Job drawing, mm, ordinate dimensions from the low corner. One solid piece. A direction names the side the tool comes from. Coordinates: 2 decimals unless noted, no trailing zeros. Loops run counter-clockwise (first coordinate to the right, second up) from the corner with the lowest first, then second, coordinate; pieces in that order, holes last. Notation, with made-up numbers: (22, -14) - (53, -14) arc R20 ccw to (53, 23) - close; hole circle Ø1 at (7, 36.25). An arc over 180 degrees is marked (long way). Use a Markdown table: item, result. Add a question column.
1. Band-saw the part on B-B, the plane z = 3.75. Give the cut face in (x, y) (1 decimal), plus the area to 3 significant figures.
2. Band-saw the part on C-C, the plane x = 20.25. Give the cut face in (y, z).
3. Wall check: probe 1 along X at (y, z) = (12, 3); probe 2 along Y at (x, z) = (2, 1.5); probe 3 along Y at (x, z) = (27, 8.5). Give the ranges that are in metal, low to high. Write a range as [from, to].
4. Band-saw the part on A-A, the plane y = 39. Give the cut face in (x, z).
5. 3-axis set-ups, long thin cutter, end or side, ignore diameter. For the marked faces 1 and 2: which of +Z, -Z, +X, -X, +Y, -Y reach the whole face in a straight line?
6. Drop flat-ended pins along their axis: pin 1 (0.9 mm diameter, centred on x = 25, z = 3, fed in from -Y); pin 2 (1 mm diameter, centred on y = 54, z = 6.5, fed in from -X); pin 3 (1.6 mm diameter, centred on x = 21.5, y = 54, fed in from +Z). Give the stop position or say it passes through.
7. Band-saw the part on D-D, the plane x = 9.5. Give the cut face in (y, z), plus the area to 3 significant figures.
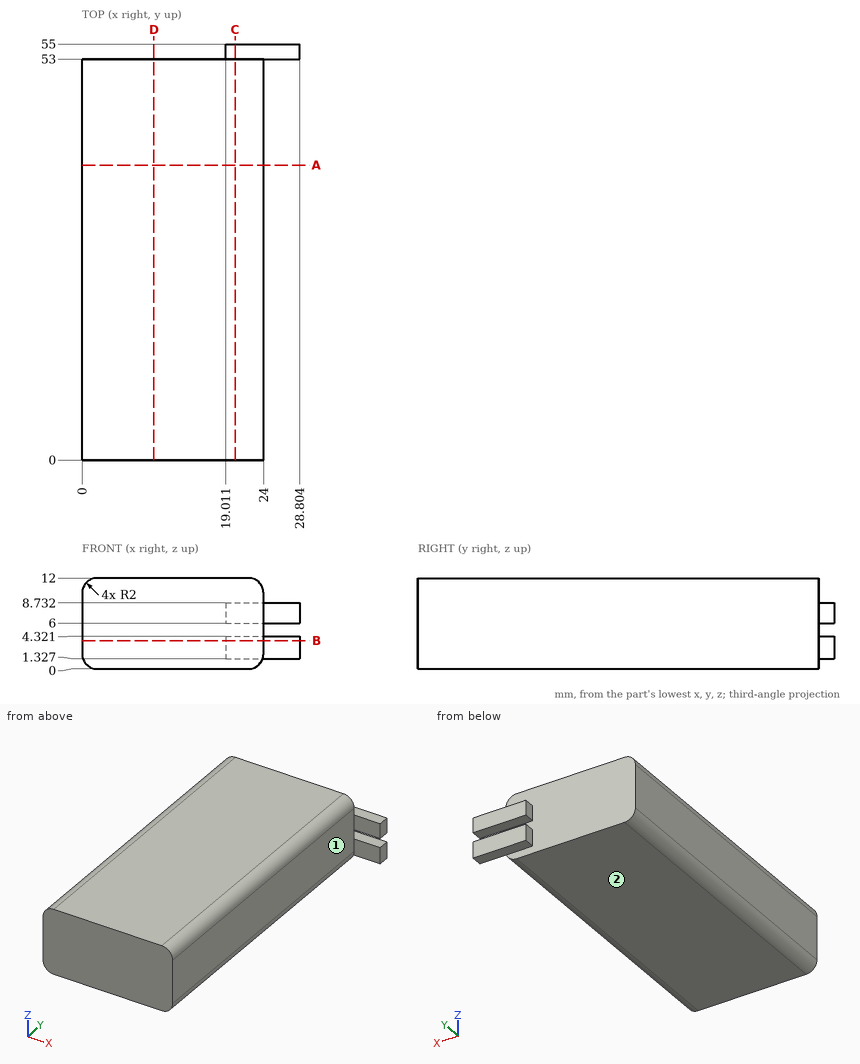
Geometry check:
| question | item | result |
|---|---|---|
| 1 | outline | (0, 0) - (24, 0) - (24, 53) - (28.8, 53) - (28.8, 55) - (19, 55) - (19, 53) - (0, 53) - close |
| 1 | area | 1,290 mm^2 |
| 2 | outline | (0, 0) - (53, 0) - (53, 1.33) - (55, 1.33) - (55, 4.32) - (53, 4.32) - (53, 6) - (55, 6) - (55, 8.73) - (53, 8.73) - (53, 12) - (0, 12) - close |
| 3 | probe 1 | x = [0, 24] |
| 3 | probe 2 | y = [0, 53] |
| 3 | probe 3 | y = [53, 55] |
| 4 | outline | (0, 2) arc R2 ccw to (2, 0) - (22, 0) arc R2 ccw to (24, 2) - (24, 10) arc R2 ccw to (22, 12) - (2, 12) arc R2 ccw to (0, 10) - close |
| 5 | face 1 | +Z, -Z, +X, -Y |
| 5 | face 2 | -Z, +X, -X, +Y, -Y |
| 6 | pin 1 | stops at y = 53 |
| 6 | pin 2 | stops at x = 19.01 |
| 6 | pin 3 | stops at z = 8.73 |
| 7 | outline | (0, 0) - (53, 0) - (53, 12) - (0, 12) - close |
| 7 | area | 636 mm^2 |
